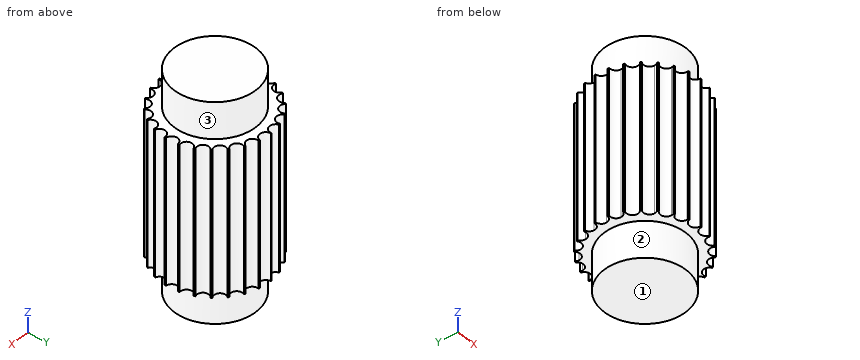
```python
from build123d import *

# Parameters (mm, degrees)
F2_DEPTH      = 101.6
F3_R          = 28.575
F4_DEPTH      = 25.4
F4_DEPTH_BACK = 127


# Not quite as in the source:
# - a variable given as a bare number and used for a length is read in inches; the dataset says mm whatever the document's units were


with BuildPart() as f2:
    # F1 (on Top) → F2 (new body)
    with BuildSketch(Plane.XY):
        with BuildLine():
            ThreePointArc((38.0275754542, -2.3480854065), (33.9582141815, 1.5680199369), (37.6493768268, 5.8424673345))
            ThreePointArc((37.6493768268, 5.8424673345), (37.5682491535, 6.3432369925), (37.4804611085, 6.8428820754))
            ThreePointArc((37.4804611085, 6.8428820754), (32.5904927394, 9.6684424763), (35.1484807634, 14.703547192))
            ThreePointArc((35.1484807634, 14.703547192), (34.949592771, 15.1702328637), (34.7445086614, 15.6342290466))
            ThreePointArc((34.7445086614, 15.6342290466), (29.3195046315, 17.2042333476), (30.5949329549, 22.705948064))
            ThreePointArc((30.5949329549, 22.705948064), (30.2898995917, 23.1112955656), (29.9794962155, 23.5125457292))
            ThreePointArc((29.9794962155, 23.5125457292), (24.3362737456, 23.7353065516), (24.254658063, 29.3823341865))
            ThreePointArc((24.254658063, 29.3823341865), (23.861293108, 29.7026714491), (23.4636978498, 30.0177428068))
            ThreePointArc((23.4636978498, 30.0177428068), (17.9318179962, 28.8802510423), (16.4979246183, 34.3428083198))
            ThreePointArc((16.4979246183, 34.3428083198), (16.0392003661, 34.5594278254), (15.5776325681, 34.7699203849))
            ThreePointArc((15.5776325681, 34.7699203849), (10.4801540403, 32.3386049206), (7.7777215434, 37.2976815311))
            ThreePointArc((7.7777215434, 37.2976815311), (7.2804272356, 37.3979328208), (6.7818422008, 37.4915539337))
            ThreePointArc((6.7818422008, 37.4915539337), (2.4164549121, 33.9084022415), (-1.3966961475, 38.0743908667))
            ThreePointArc((-1.3966961475, 38.0743908667), (-1.611243941, 38.0659151074), (-1.8257405619, 38.0562303887))
            ThreePointArc((-1.8257405619, 38.0562303887), (-1.8097889216, 37.8477980327), (-1.8044671093, 37.638823919))
            ThreePointArc((-1.8044671093, 37.638823919), (-5.4804796414, 33.5557575077), (-9.9257732847, 36.7843584245))
            ThreePointArc((-9.9257732847, 36.7843584245), (-10.4146635829, 36.648939718), (-10.901707494, 36.5070236217))
            ThreePointArc((-10.901707494, 36.5070236217), (-10.7216553993, 35.8248982817), (-10.661041443, 35.1220187156))
            ThreePointArc((-10.661041443, 35.1220187156), (-13.8468450451, 31.1207754191), (-18.4601131844, 33.3291797262))
            ThreePointArc((-18.4601131844, 33.3291797262), (-18.9022425388, 33.0804357137), (-19.3410207665, 32.8258269616))
            ThreePointArc((-19.3410207665, 32.8258269616), (-18.8304314471, 31.7405924789), (-18.6552519207, 30.5541071359))
            ThreePointArc((-18.6552519207, 30.5541071359), (-21.3643249191, 26.6933193437), (-25.9163927322, 27.9275954524))
            ThreePointArc((-25.9163927322, 27.9275954524), (-26.2859410341, 27.580052646), (-26.6508291737, 27.2276202478))
            ThreePointArc((-26.6508291737, 27.2276202478), (-25.6675808238, 25.8545575842), (-25.3202410927, 24.2018526781))
            ThreePointArc((-25.3202410927, 24.2018526781), (-27.5730476059, 20.5380946086), (-31.8591693457, 20.8950551232))
            ThreePointArc((-31.8591693457, 20.8950551232), (-32.1345551797, 20.4690098296), (-32.4042439666, 20.0393356415))
            ThreePointArc((-32.4042439666, 20.0393356415), (-30.8413491085, 18.5309299599), (-30.266777295, 16.4362234724))
            ThreePointArc((-30.266777295, 16.4362234724), (-32.090467362, 13.0231821609), (-35.9413881732, 12.6422551859))
            ThreePointArc((-35.9413881732, 12.6422551859), (-36.1065291595, 12.1625882135), (-36.2652689185, 11.6807649693))
            ThreePointArc((-36.2652689185, 11.6807649693), (-34.0595315808, 10.2167411474), (-33.2059855622, 7.7107279494))
            ThreePointArc((-33.2059855622, 7.7107279494), (-34.633997298, 4.5984165422), (-37.9246499035, 3.6511545708))
            ThreePointArc((-37.9246499035, 3.6511545708), (-37.9699019004, 3.1458782044), (-38.0084223177, 2.6400441138))
            ThreePointArc((-38.0084223177, 2.6400441138), (-35.1463921507, 1.415528136), (-33.9662177648, -1.4650698011))
            ThreePointArc((-33.9662177648, -1.4650698011), (-35.0377873736, -4.231044916), (-37.6931331536, -5.5531714423))
            ThreePointArc((-37.6931331536, -5.5531714423), (-37.6158534696, -6.0545493438), (-37.5319049742, -6.554853851))
            ThreePointArc((-37.5319049742, -6.554853851), (-34.0527474172, -7.3423365778), (-32.5030767644, -10.5553082894))
            ThreePointArc((-32.5030767644, -10.5553082894), (-33.2626635907, -12.9344157776), (-35.2603583731, -14.4331953289))
            ThreePointArc((-35.2603583731, -14.4331953289), (-35.0650600987, -14.9013945747), (-34.8635452362, -15.3669519932))
            ThreePointArc((-34.8635452362, -15.3669519932), (-30.8586295725, -15.530858571), (-28.9020091826, -19.029122639))
            ThreePointArc((-28.9020091826, -19.029122639), (-29.3986442237, -20.9865001474), (-30.7683982573, -22.4703286287))
            ThreePointArc((-30.7683982573, -22.4703286287), (-30.4664867033, -22.878006643), (-30.1591738296, -23.2816286783))
            ThreePointArc((-30.1591738296, -23.2816286783), (-25.7683757069, -22.6593523381), (-23.373315365, -26.3916468007))
            ThreePointArc((-23.373315365, -26.3916468007), (-23.6598827933, -27.8986118146), (-24.4795807808, -29.1952072231))
            ThreePointArc((-24.4795807808, -29.1952072231), (-24.0886874142, -29.5185558363), (-23.6935234304, -29.8366711859))
            ThreePointArc((-23.6935234304, -29.8366711859), (-19.0984337687, -28.3012799336), (-16.2398679583, -32.2129134548))
            ThreePointArc((-16.2398679583, -32.2129134548), (-16.3723301811, -33.2473835979), (-16.7611693897, -34.2151019389))
            ThreePointArc((-16.7611693897, -34.2151019389), (-16.3041221659, -34.4352377718), (-15.844184429, -34.649268676))
            ThreePointArc((-15.844184429, -34.649268676), (-11.2586011252, -32.1193105722), (-7.9182563272, -36.1529638633))
            ThreePointArc((-7.9182563272, -36.1529638633), (-7.9548339389, -36.6997804834), (-8.0639150202, -37.2368537144))
            ThreePointArc((-8.0639150202, -37.2368537144), (-7.567405243, -37.3409209566), (-7.0695538613, -37.4383681295))
            ThreePointArc((-7.0695538613, -37.4383681295), (-2.7277955027, -33.8851355215), (1.1055420333, -37.9817012719))
            ThreePointArc((1.1055420333, -37.9817012719), (1.105223389, -38.0328515683), (1.1042675055, -38.083993925))
            ThreePointArc((1.1042675055, -38.083993925), (1.611243941, -38.0659151074), (2.1179347234, -38.0410876883))
            ThreePointArc((2.1179347234, -38.0410876883), (5.5309497632, -33.5414309717), (10.2079614225, -36.707050053))
            ThreePointArc((10.2079614225, -36.707050053), (10.6957973741, -36.5678809686), (11.1817370971, -36.4222288649))
            ThreePointArc((11.1817370971, -36.4222288649), (13.4156740687, -31.2352154819), (18.7155160648, -33.1864348556))
            ThreePointArc((18.7155160648, -33.1864348556), (19.1557221841, -32.9343029015), (19.592532238, -32.6763321152))
            ThreePointArc((19.592532238, -32.6763321152), (20.5169304634, -27.1048807648), (26.1300949689, -27.7277503039))
            ThreePointArc((26.1300949689, -27.7277503039), (26.4969634631, -27.377379846), (26.8591343834, -27.0221557277))
            ThreePointArc((26.8591343834, -27.0221557277), (26.4200095201, -21.3916360729), (32.018690847, -20.6497805423))
            ThreePointArc((32.018690847, -20.6497805423), (32.2907967999, -20.2216330208), (32.5571780061, -19.7899004616))
            ThreePointArc((32.5571780061, -19.7899004616), (30.780174702, -14.4291317214), (36.0374129719, -12.3658750718))
            ThreePointArc((36.0374129719, -12.3658750718), (36.1988655471, -11.8849540641), (36.3539005248, -11.4019260055))
            ThreePointArc((36.3539005248, -11.4019260055), (33.3427947854, -6.6239740954), (37.9515702047, -3.3598093687))
            ThreePointArc((37.9515702047, -3.3598093687), (37.9929406615, -2.8542003943), (38.0275754542, -2.3480854065))
        make_face()
    extrude(amount=F2_DEPTH)

    # F3 (on face) → F4 (join, two sides)
    with BuildSketch(Plane(origin=(0, 0, 0), x_dir=(1, 0, 0), z_dir=(0, 0, -1))) as f4_sk:
        Circle(F3_R)
    extrude(amount=F4_DEPTH)
    extrude(f4_sk.sketch, amount=-F4_DEPTH_BACK)


solid = f2.part
```
Geometry check sheet. Reference: the model listing, model coordinates, mm. Face numbers are marked on the shaded views. A direction names the side the tool comes from. Give positions to 0.01 mm unless a question says otherwise; leave off trailing zeros. Loops run counter-clockwise (first coordinate to the right, second up) from the corner with the lowest first, then second, coordinate; pieces in that order, holes last. Notation, with made-up numbers: M 61,86 L 67,86 A25 ccw 67,110 Z; hole C -37,-27.5 d5. An arc over 180 degrees is marked long. Answer as CSV lines item,"result".
Item 1: Access from +Z, -Z, +X, -X, +Y, -Y to the whole of each face (thin tool, end or side, straight path). Record for the marked faces 1, 2 and 3.
Values:
face 1,"-Z, +X, -X, +Y, -Y"
face 2,"-Z"
face 3,"+Z"
Item 2: Material ranges on line 1 (X direction, y = 3.5, z = 93); line 2 (Z direction, x = -26, y = 18.5); line 3 (X direction, y = -23, z = 98.5), recorded low to high.
Values:
line 1,"x = -37.94 to 34.34"
line 2,"z = 0 to 101.6"
line 3,"x = -30.37 to -29.79, -25.17 to 25.62"
Item 3: Cross-section at A-A on x = -3.5. Record the cut outline in (y, z).
Values:
outline,"M -33.91,0 L -28.36,0 L -28.36,-25.4 L 28.36,-25.4 L 28.36,0 L 34.32,0 L 34.32,101.6 L 28.36,101.6 L 28.36,127 L -28.36,127 L -28.36,101.6 L -33.91,101.6 Z"
Item 4: Depth check by flat-ended pin: P1, Ø1.5, axis at x = 26, z = 3.5, coming from the +Y side; P2, Ø12, axis at y = 23, z = 8.5, coming from the +X side; P3, Ø3, axis at y = 13, z = 33, coming from the +X side; P4, Ø6, axis at x = -29, y = 1.5, coming from the -Z side. Enter the tip coordinate at first touch or a pass-through.
Values:
P1,"stops at y = 23.03"
P2,"stops at x = 30.59"
P3,"stops at x = 34.67"
P4,"stops at z = -25.4"
Item 5: Cross-section at B-B on x = -21. Record the cut outline in (y, z), and give its area (3 significant figures).
Values:
outline,"M -28.16,0 L -19.38,0 L -19.38,-25.4 L 19.38,-25.4 L 19.38,0 L 26.85,0 L 26.85,101.6 L 19.38,101.6 L 19.38,127 L -19.38,127 L -19.38,101.6 L -28.16,101.6 Z"
area,"7,560 mm²"
